The model under review builds one solid part; all positions refer to its coordinate system, in mm. Face numbers are marked on the shaded views. A direction names the side the tool comes from. Coordinates: 2 decimals unless noted, no trailing zeros. Loops run counter-clockwise (first coordinate to the right, second up) from the corner with the lowest first, then second, coordinate; pieces in that order, holes last. Notation, with made-up numbers: M 69,58.5 L 108,58.5 A25 ccw 108,76.5 Z; hole C 32.5,66.25 d6. An arc over 180 degrees is marked long. Write item = value, one per line. Start each with the question number.
Q1. Clearance check with a flat-ended pin moving along its axis: pin 1 Ø2.5 at (y, z) = (1, 5) entering from +X. State where the tip first meets the part, or that it passes through.
Q2. Wall thickness on probe 1 along X at (y, z) = (1, 8.75); probe 2 along Y at (x, z) = (0.25, 12); probe 3 along X at (y, z) = (-7, 22.5): over which ranges is each line inside the solid? List them lowest first.
Q3. Mouldability with a two-part tool opening along X and no side actions: class the marked faces 3, 4, 5 and 6 as released by +X, released by -X, zero draft, split by the parting line, or undercut.
Q4. For the marked faces 1 and 2, list the 3-axis set-ups (+Z, -Z, +X, -X, +Y, -Y) from which the entire face can be reached by the end or side of a thin tool; tool diameter is ignored.
Q5. We need section C-C on z = 22.5. Give the boundary of the cut face in (x, y), and give its area (3 significant figures).
Q6. We need section D-D on x = -4. Give the boundary of the cut face in (y, z), and give its area (3 significant figures).
Q7. We need section A-A on y = 1. Give the boundary of the cut face in (x, z), and give its area (3 significant figures).
Q8. We need section B-B on x = 0. Give the boundary of the cut face in (y, z), and give its area (3 significant figures).
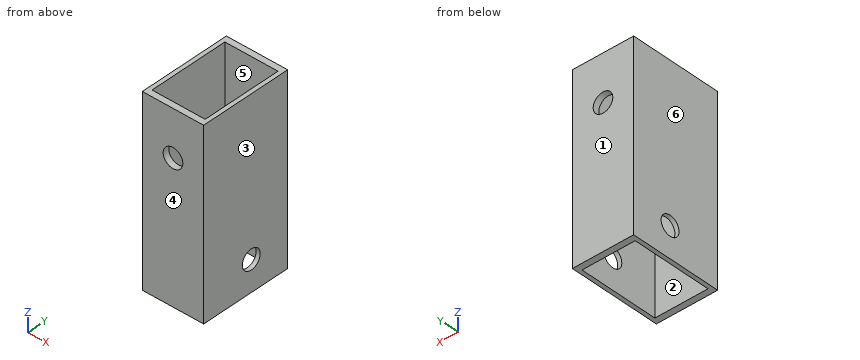
from build123d import *

# Parameters (mm, degrees)
SKETCH_1_W          = 10
SKETCH_1_H          = 15
SKETCH_1_W_2        = 8.666666666
SKETCH_1_H_2        = 13
EXTRUDE_1_DEPTH     = 30
SKETCH_3_R          = 1.6
CUT_EXTRUDE_2_DEPTH = 34.911649916
SKETCH_4_R          = 1.6
CUT_EXTRUDE_3_DEPTH = 33.5


with BuildPart() as part:
    # ｽｹｯﾁ1 → ﾎﾞｽ - 押し出し1 (new body)
    with BuildSketch(Plane.XY):
        Rectangle(SKETCH_1_W, SKETCH_1_H)
        Rectangle(SKETCH_1_W_2, SKETCH_1_H_2, mode=Mode.SUBTRACT)
    extrude(amount=EXTRUDE_1_DEPTH)

    # ｽｹｯﾁ3 → ｶｯﾄ - 押し出し2 (cut, through all)
    with BuildSketch(Plane(origin=(0, 7.5, 0), x_dir=(1, 0, 0), z_dir=(0, 1, 0))):
        with Locations(Location((0, -22.5, 0), (0, 0, 270))):
            Circle(SKETCH_3_R)
    extrude(amount=-CUT_EXTRUDE_2_DEPTH, mode=Mode.SUBTRACT)

    # ｽｹｯﾁ4 → ｶｯﾄ - 押し出し3 (cut, through all)
    with BuildSketch(Plane.ZY.offset(5)):
        with Locations((5, 1)):
            Circle(SKETCH_4_R)
    extrude(amount=-CUT_EXTRUDE_3_DEPTH, mode=Mode.SUBTRACT)


solid = part.part
Returned:
q1.pin_1 = through
q2.probe_1 = -5 to -4.33, 4.33 to 5
q2.probe_2 = -7.5 to -6.5, 6.5 to 7.5
q2.probe_3 = -5 to -1.6, 1.6 to 5
q3.face_3 = released by +X
q3.face_4 = zero draft
q3.face_5 = undercut
q3.face_6 = released by -X
q4.face_1 = +Z, -Z, +X, -X, +Y
q4.face_2 = +Z, -Z
q5.outline = M -5,-7.5 L -1.6,-7.5 L -1.6,-6.5 L -4.33,-6.5 L -4.33,6.5 L -1.6,6.5 L -1.6,7.5 L -5,7.5 Z; M 1.6,-7.5 L 5,-7.5 L 5,7.5 L 1.6,7.5 L 1.6,6.5 L 4.33,6.5 L 4.33,-6.5 L 1.6,-6.5 Z
q5.area = 30.9 mm^2
q6.outline = M -7.5,0 L -6.5,0 L -6.5,30 L -7.5,30 Z; M 6.5,0 L 7.5,0 L 7.5,30 L 6.5,30 Z
q6.area = 60.0 mm^2
q7.outline = M -5,0 L -4.33,0 L -4.33,3.4 L -5,3.4 Z; M -5,6.6 L -4.33,6.6 L -4.33,30 L -5,30 Z; M 4.33,0 L 5,0 L 5,3.4 L 4.33,3.4 Z; M 4.33,6.6 L 5,6.6 L 5,30 L 4.33,30 Z
q7.area = 35.7 mm^2
q8.outline = M -7.5,0 L -6.5,0 L -6.5,20.9 L -7.5,20.9 Z; M -7.5,24.1 L -6.5,24.1 L -6.5,30 L -7.5,30 Z; M 6.5,0 L 7.5,0 L 7.5,20.9 L 6.5,20.9 Z; M 6.5,24.1 L 7.5,24.1 L 7.5,30 L 6.5,30 Z
q8.area = 53.6 mm^2
